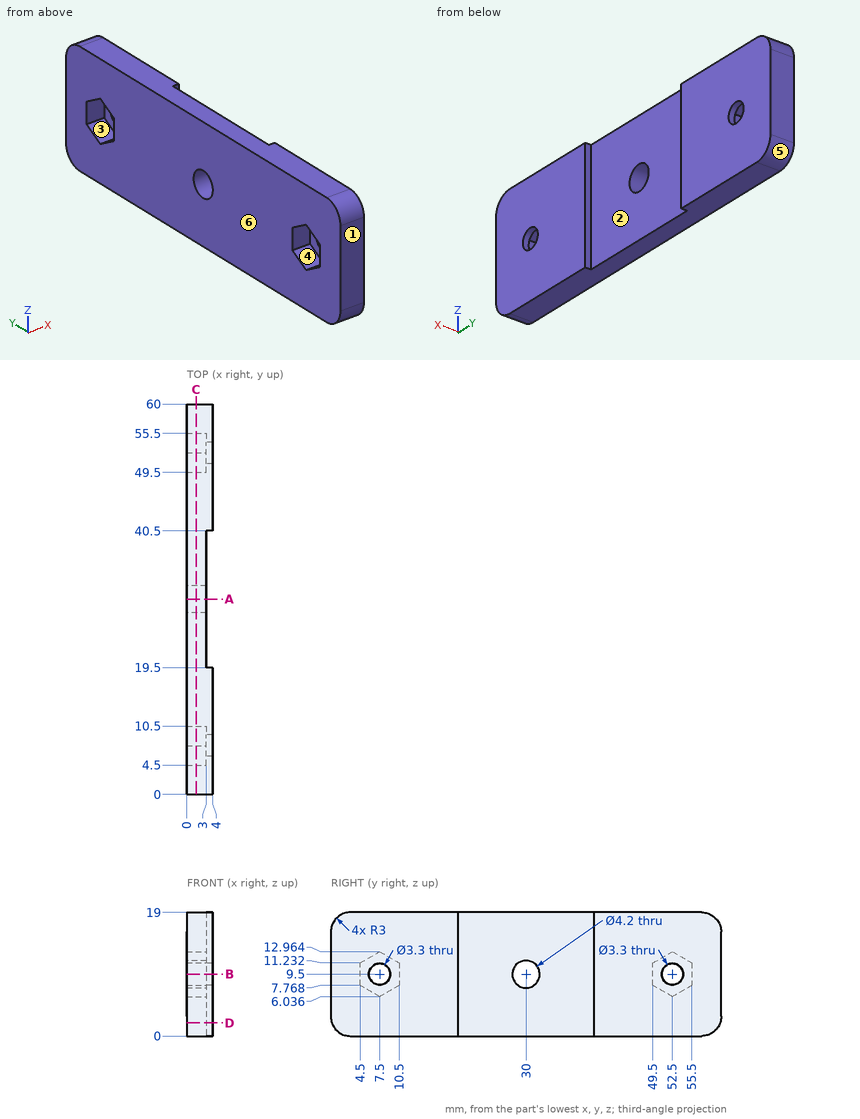
Check sheet for the drawn part. Datum: minimum x, y, z corner. Units: mm. A direction names the side the tool comes from. Round coordinates to 2 decimals unless told otherwise and drop trailing zeros. Loops run counter-clockwise (first coordinate to the right, second up) from the corner with the lowest first, then second, coordinate; pieces in that order, holes last.
Item 1: Mould release check, pull along Y, two halves, no side actions. Record for the marked faces 4, 5 and 6: pulls with the +Y half, pulls with the -Y half, needs draft (parallel to the pull), parting line crosses it, or undercut.
Item 2: Cross-section at D-D on z = 2. Record the boundary of the cut face in (x, y), then the cut area to 3 significant figures.
Item 3: Thickness scan on line 1 (Y direction, x = 0.75, z = 9.5); line 2 (Y direction, x = 3.85, z = 9.5); line 3 (Y direction, x = 1.85, z = 11.75). Record the ranges inside material, lowest first.
Item 4: Cross-section at B-B on z = 9.5. Record the boundary of the cut face in (x, y), then the cut area to 3 significant figures.
Item 5: Cross-section at A-A on y = 30. Record the boundary of the cut face in (x, z), then the cut area to 3 significant figures.
Item 6: Access from +Z, -Z, +X, -X, +Y, -Y to the whole of each face (thin tool, end or side, straight path). Record for the marked faces 1, 2 and 3.
Item 7: Cross-section at C-C on x = 1.45. Record the boundary of the cut face in (y, z), then the cut area to 3 significant figures.
Item 8: Gauge pin test, flat ends, axial feed: pin 1 (3 mm diameter, centred on y = 52.5, z = 9.5, fed in from -X); pin 2 (3 mm diameter, centred on y = 53, z = 9.5, fed in from -X). Record the tip position at first contact, or that the pin passes through.
Answer sheet:
1. face 4: undercut
1. face 5: pulls with the +Y half
1. face 6: needs draft
2. outline: (0, 0.17) - (4, 0.17) - (4, 19.5) - (3, 19.5) - (3, 40.5) - (4, 40.5) - (4, 59.83) - (0, 59.83) - close
2. area: 218 mm2
3. line 1: y = 0 to 4.5, 10.5 to 27.9, 32.1 to 49.5, 55.5 to 60
3. line 2: y = 0 to 5.85, 9.15 to 19.5, 40.5 to 50.85, 54.15 to 60
3. line 3: y = 0 to 5.4, 9.6 to 50.4, 54.6 to 60
4. outline: (0, 0) - (4, 0) - (4, 5.85) - (3, 5.85) - (3, 4.5) - (0, 4.5) - close; (0, 10.5) - (3, 10.5) - (3, 9.15) - (4, 9.15) - (4, 19.5) - (3, 19.5) - (3, 27.9) - (0, 27.9) - close; (0, 32.1) - (3, 32.1) - (3, 40.5) - (4, 40.5) - (4, 50.85) - (3, 50.85) - (3, 49.5) - (0, 49.5) - close; (0, 55.5) - (3, 55.5) - (3, 54.15) - (4, 54.15) - (4, 60) - (0, 60) - close
4. area: 164 mm2
5. outline: (0, 0) - (3, 0) - (3, 7.4) - (0, 7.4) - close; (0, 11.6) - (3, 11.6) - (3, 19) - (0, 19) - close
5. area: 44.4 mm2
6. face 1: +Z, -Z, +X, -X, -Y
6. face 2: +Z, -Z, +X
6. face 3: -X
7. outline: (0, 3) arc R3 ccw to (3, 0) - (57, 0) arc R3 ccw to (60, 3) - (60, 16) arc R3 ccw to (57, 19) - (3, 19) arc R3 ccw to (0, 16) - close; hole (4.5, 7.77) - (7.5, 6.04) - (10.5, 7.77) - (10.5, 11.23) - (7.5, 12.96) - (4.5, 11.23) - close; hole circle Ø4.2 at (30, 9.5); hole (49.5, 7.77) - (52.5, 6.04) - (55.5, 7.77) - (55.5, 11.23) - (52.5, 12.96) - (49.5, 11.23) - close
7. area: 1,060 mm2
8. pin 1: passes through
8. pin 2: stops at x = 3
